Build history of the part. All positions in model axes, mm. A direction names the side the tool comes from. Coordinates: 2 decimals unless noted, no trailing zeros. Order: outer loops, then holes, each group sorted by start corner. A loop starts at its lowest first (then second) coordinate and runs counter-clockwise, first axis right, second up. Notation, with made-up numbers: (-3, 73) - (33, 73) arc R16 ccw to (33, 84) - close; hole circle Ø3 at (17.25, 21.5). An arc over 180 degrees is marked (long way). Write each question's results on one line, items separated by ' | '.
Autodesk Inventor part; units mm, degrees
ref_plane "Work Plane1" through (-3, 0, 31) normal (0, 0, -1) x (0, 1, 0)
ref_plane "YZ Plane" through (0, 0, 0) normal (1, 0, 0) x (0, 1, 0)
ref_plane "XZ Plane" through (0, 0, 0) normal (0, 1, 0) x (-1, 0, 0)
sketch "Sketch1" plane through (0, 0, 0) normal (0, 0, 1) x (1, 0, 0)
  line L0 (0, 20) -> (0, 0)
  line L1 (0, 20) -> (-3, 20)
  line L2 (-3, 0) -> (-3, 20)
  line L3 (0, 0) -> (-3, 0)
  arc A0 (-3, 20) -> (-9.8284, 20) centre (-6.4142, 20) ccw
  circle A1 centre (-6.4142, 20) radius 6.4142
  line L4 (-9.8284, 20) -> (-12.8284, 20)
  line L5 (-12.8284, 20) -> (-12.8284, 0)
  line L6 (-12.8284, 0) -> (-9.8284, 0)
  line L7 (-9.8284, 0) -> (-9.8284, 20)
  point P0 (-3, 14.57)
ref_plane "Work Plane1" through (-3, 0, 31) normal (0, 0, -1) x (0, 1, 0)
extrude "Extrusion1" add sketch "Sketch1" along normal up to surface (31 mm away) contours A1 L2 L1 | L1 A0 L4 A1 | L0 L3 L2 A1 | L4 L7 A1 | A1 L7 L6 L5
sketch "Sketch2" plane through (-12.8284, 0, 0) normal (-1, 0, 0) x (0, 0, 1)
  line L0 (0, 0) -> (31, 0)
  line L1 (15.5, 0) -> (15.5, 20)
  line L2 (0, 20) -> (31, 20)
  line L3 (15.5, 10) -> (4.5, 10)
  line L4 (15.5, 10) -> (26.5, 10)
  line L5 (26.5, 10) -> (26.5, 5)
  line L6 (4.5, 10) -> (4.5, 15)
  circle A0 centre (26.5, 5) radius 1.5
  circle A1 centre (4.5, 15) radius 1.5
  line L7 (26.5, 5) -> (4.5, 5)
  line L8 (4.5, 5) -> (4.5, 15)
  line L9 (4.5, 15) -> (26.5, 15)
  line L10 (26.5, 15) -> (26.5, 5)
  circle A2 centre (4.5, 5) radius 1.5
  circle A3 centre (26.5, 15) radius 1.5
  dimension "d2" = 11
  dimension "d3" = 11
  dimension "d4" = 5
  dimension "d5" = 5
  dimension "d6" = 3
  dimension "d7" = 3
  dimension "d8" = 3
  dimension "d9" = 3
extrude "Extrusion2" cut sketch "Sketch2" against normal up to surface (3 mm away) contours L7 L5 A0 | A0 L5 L7 | A2 L8 L7 | L7 L8 A2 | L9 L6 A1 | A1 L6 L9 | A3 L10 L9 | L9 L10 A3
properties part number "back_helmet_holder" material "Stainless Steel"
1. Drop flat-ended pins along their axis: pin 1 Ø2.5 at (y, z) = (15, 4.5) entering from -X; pin 2 Ø3 at (x, z) = (-7.5, 17.5) entering from -Y; pin 3 Ø1 at (y, z) = (23, 24.5) entering from -X. Give the stop position or say it passes through.
Solved:
pin 1: stops at x = -3 | pin 2: stops at y = 22.23 | pin 3: stops at x = -12.32
2. Band-saw the part on B-B on z = 4.5. Give the cut face in (x, y).
Solved:
outline: (-12.83, 0) - (-9.83, 0) - (-9.83, 3.5) - (-12.83, 3.5) - close; (-12.83, 6.5) - (-9.83, 6.5) - (-9.83, 13.5) - (-12.83, 13.5) - close; (-12.83, 16.5) - (-9.83, 16.5) - (-9.83, 20) arc R3.41 cw to (-3, 20) - (-3, 0) - (0, 0) - (0, 20) arc R6.41 ccw to (-12.83, 20) - close
3. Band-saw the part on D-D on y = 22.25. Give the cut face in (x, z).
Solved:
outline: (-12.42, 0) - (-8.98, 0) - (-8.98, 31) - (-12.42, 31) - close; (-3.85, 0) - (-0.41, 0) - (-0.41, 31) - (-3.85, 31) - close
4. Band-saw the part on A-A on y = 10.5. Give the cut face in (x, z).
Solved:
outline: (-12.83, 0) - (-9.83, 0) - (-9.83, 31) - (-12.83, 31) - close; (-3, 0) - (0, 0) - (0, 31) - (-3, 31) - close
5. Band-saw the part on C-C on y = 15. Give the cut face in (x, z).
Solved:
outline: (-12.83, 0) - (-9.83, 0) - (-9.83, 3) - (-12.83, 3) - close; (-12.83, 6) - (-9.83, 6) - (-9.83, 25) - (-12.83, 25) - close; (-12.83, 28) - (-9.83, 28) - (-9.83, 31) - (-12.83, 31) - close; (-3, 0) - (0, 0) - (0, 31) - (-3, 31) - close
6. Probe line 1 (Z direction, x = -11.6, y = 5); line 2 (X direction, y = 16.5, z = 24.5); line 3 (Y direction, x = -11.1, z = 4.5). List the from-to ranges inside material, lowest first.
Solved:
line 1: z = 0 to 3, 6 to 25, 28 to 31 | line 2: x = -12.83 to -9.83, -3 to 0 | line 3: y = 0 to 3.5, 6.5 to 13.5, 16.5 to 24.38
7. Tool access for faces 1 (the face through (-9.828, 10, 15)), 2 (the face through (0, 10, 15)), 3 (the face through (-11, 15, 25)): list every direction of +Z, -Z, +X, -X, +Y, -Y with a clear straight run to the whole face (end or side of a thin tool).
Solved:
face 1: +Z, -Z, -Y | face 2: +Z, -Z, +X, +Y, -Y | face 3: -X
8. Two-plate mould, pull along Z, no slides. Class faces 4 (the face through (-11.349, 14.425, 5.886)), 5 (the face through (-2, 13, 31)), 6 (the face through (-12.828, 10, 15)): +Z half, -Z half, draft (parallel to the pull), parting line (faces both ways), or undercut.
Solved:
face 4: undercut | face 5: +Z half | face 6: draft
